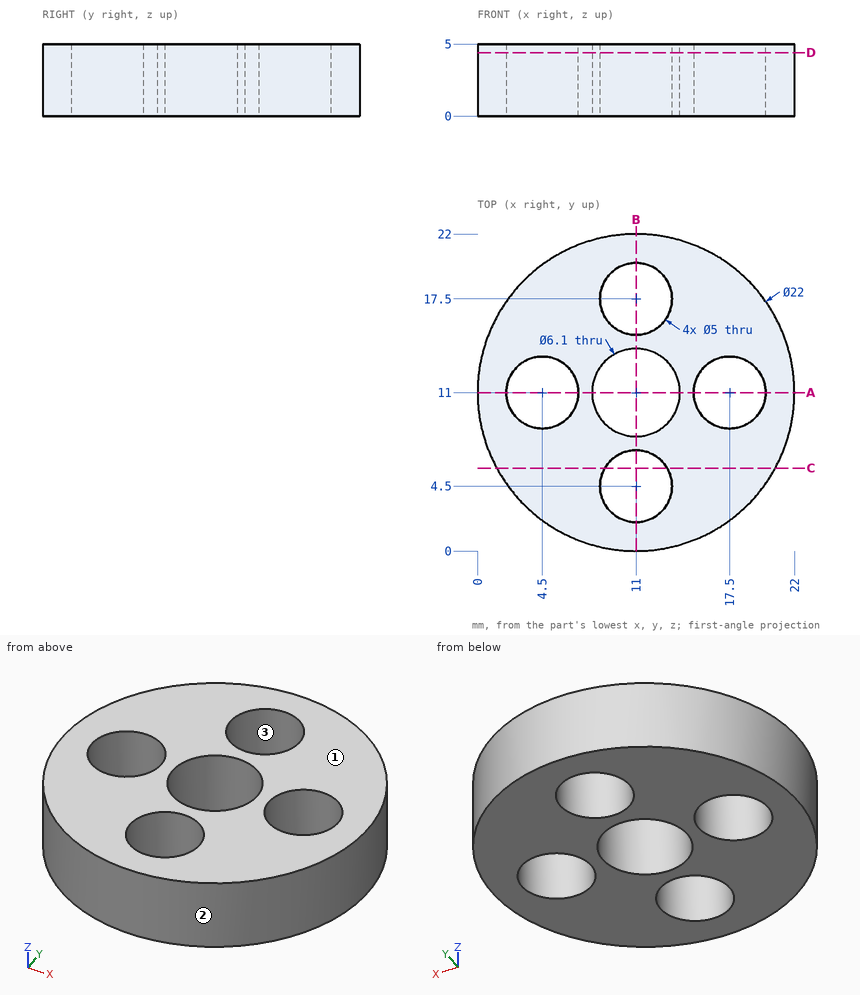
Source: three-view drawing plus pictorial views. Frame: mm from the lowest corner of the part. Coordinates: 2 decimals unless noted, no trailing zeros. Order: outer loops, then holes, each group sorted by start corner. A loop starts at its lowest first (then second) coordinate and runs counter-clockwise, first axis right, second up. Notation, with made-up numbers: M 9,-12 L 68,-12 A20 cw 68,4 Z; hole C 2,51 d4. An arc over 180 degrees is marked long. Answer in a Markdown table with one row per item.
(1) Draft query along Y for the marked faces 1, 2 and 3. Return one class per face: pulls with the +Y half, pulls with the -Y half, needs draft (parallel to the pull), parting line crosses it, or undercut.
Numbers:
| item | result |
|---|---|
| face 1 | needs draft |
| face 2 | parting line crosses it |
| face 3 | undercut |
(2) Section query C-C, the plane y = 5.75. Output: boundary loops of the cut face in (x, z).
Numbers:
| item | result |
|---|---|
| outline | M 1.33,0 L 8.83,0 L 8.83,5 L 1.33,5 Z; M 13.17,0 L 20.67,0 L 20.67,5 L 13.17,5 Z |
(3) Section query D-D, the plane z = 4.4. Output: boundary loops of the cut face in (x, y).
Numbers:
| item | result |
|---|---|
| outline | C 11,11 d22; hole C 4.5,11 d5; hole C 11,11 d6.1; hole C 11,4.5 d5; hole C 11,17.5 d5; hole C 17.5,11 d5 |
(4) Section query A-A, the plane y = 11. Output: boundary loops of the cut face in (x, z).
Numbers:
| item | result |
|---|---|
| outline | M 0,0 L 2,0 L 2,5 L 0,5 Z; M 7,0 L 7.95,0 L 7.95,5 L 7,5 Z; M 14.05,0 L 15,0 L 15,5 L 14.05,5 Z; M 20,0 L 22,0 L 22,5 L 20,5 Z |
(5) Contact query for flat-ended pins moving along their axis: pin 1 Ø1 at (x, z) = (7.5, 2) entering from +Y; pin 2 Ø1 at (x, z) = (10, 2.5) entering from +Y; pin 3 Ø2 at (y, z) = (14.5, 1.5) entering from +X. Output: stop coordinate, or through.
Numbers:
| item | result |
|---|---|
| pin 1 | stops at y = 21.58 |
| pin 2 | stops at y = 21.99 |
| pin 3 | stops at x = 21.71 |
(6) Material intervals for line 1 (Y direction, x = 11, z = 2.6); line 2 (X direction, y = 10.25, z = 1.95); line 3 (Y direction, x = 12.25, z = 4.75), sorted ascending. Write a range as [from, to].
Numbers:
| item | result |
|---|---|
| line 1 | y = [0, 2], [7, 7.95], [14.05, 15], [20, 22] |
| line 2 | x = [0.03, 2.12], [6.88, 8.04], [13.96, 15.12], [19.88, 21.97] |
| line 3 | y = [0.07, 2.33], [6.67, 8.22], [13.78, 15.33], [19.67, 21.93] |
